Autodesk Inventor part; units mm, degrees
ref_plane "YZ Plane" through (0, 0, 0) normal (1, 0, 0) x (0, 1, 0)
ref_plane "XZ Plane" through (0, 0, 0) normal (0, 1, 0) x (-1, 0, 0)
ref_plane "XY Plane" through (0, 0, 0) normal (0, 0, 1) x (1, 0, 0)
sketch "Sketch1" plane through (0, 0, 0) normal (0, 0, 1) x (1, 0, 0)
  line L0 (0, 0) -> (-30, 0)
  line L1 (0, 0) -> (30, 0)
  line L2 (30, 0) -> (0, 51.9615)
  line L3 (0, 51.9615) -> (-30, 0)
  dimension "d0" = 30
  dimension "d1" = 30
  dimension "d2" = 60
  dimension "d3" = 60
extrude "Extrusion1" add sketch "Sketch1" along normal blind 12
sketch "Sketch2" plane through (0, 0, 12) normal (0, 0, 1) x (1, 0, 0)
  line L0 (0, 0) -> (0, 30)
  circle A0 centre (0, 30) radius 3
  dimension "d7" = 30
  dimension "d8" = 6
extrude "Extrusion2" cut sketch "Sketch2" against normal through all
fillet "Fillet2" radius 2 1 edges at (0, 51.9615, 6)
properties part number "Rocker Base Joint"
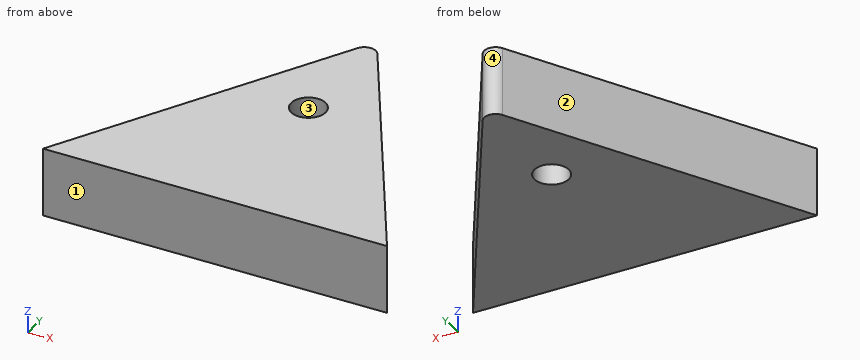
Input: part model. Units: mm. Frame: model coordinates. Face numbers are marked on the shaded views. Round coordinates to 2 decimals unless told otherwise and drop trailing zeros. Write each loop counter-clockwise with the first axis right and the second up, starting at its lowest first coordinate (ties: lowest second). Pieces come first, ordered by that corner, then holes. Notation, with made-up numbers: (-26, 89) - (5, 89) arc R21 ccw to (5, 118) - close; hole circle Ø2 at (25.5, 0.25). An arc over 180 degrees is marked (long way). Write item = value, one per line.
(1) Section query B-B on z = 1.5. Output: boundary loops of the cut face in (x, y).
Geometry check:
outline = (-30, 0) - (30, 0) - (1.73, 48.96) arc R2 ccw to (-1.73, 48.96) - close; hole circle Ø6 at (0, 30)
(2) Pull-direction query (X, two-part tool) for the marked faces 1, 2, 3 and 4; classes: +X half, -X half, draft (parallel to the pull), parting line (faces both ways), or undercut.
Geometry check:
face_1 = draft
face_2 = -X half
face_3 = undercut
face_4 = parting line
(3) Material intervals for probe 1 along X at (y, z) = (30, 8); probe 2 along X at (y, z) = (42.5, 1.5); probe 3 along X at (y, z) = (16.5, 1.75), sorted ascending.
Geometry check:
probe_1 = -12.68 to -3, 3 to 12.68
probe_2 = -5.46 to 5.46
probe_3 = -20.47 to 20.47
(4) Section query D-D on x = -18. Output: boundary loops of the cut face in (y, z).
Geometry check:
outline = (0, 0) - (20.78, 0) - (20.78, 12) - (0, 12) - close
(5) Section query A-A on x = 0. Output: boundary loops of the cut face in (y, z), then the cut area to 3 significant figures.
Geometry check:
outline = (0, 0) - (27, 0) - (27, 12) - (0, 12) - close; (33, 0) - (49.96, 0) - (49.96, 12) - (33, 12) - close
area = 528 mm^2
(6) Section query C-C on y = 30. Output: boundary loops of the cut face in (x, z), then the cut area to 3 significant figures.
Geometry check:
outline = (-12.68, 0) - (-3, 0) - (-3, 12) - (-12.68, 12) - close; (3, 0) - (12.68, 0) - (12.68, 12) - (3, 12) - close
area = 232 mm^2
(7) Contact query for flat-ended pins moving along their axis: pin 1 Ø1 at (x, z) = (-6.5, 1.5) entering from +Y; pin 2 Ø5 at (x, z) = (-18.5, 10.5) entering from +Y; pin 3 Ø5 at (y, z) = (38, 9) entering from -X. Output: stop coordinate, or through.
Geometry check:
pin_1 = 41.57
pin_2 = 24.25
pin_3 = -9.5
